from build123d import *

# Parameters (mm, degrees)
SKETCH_3_W          = 80
SKETCH_3_H          = 56
EXTRUDE_1_DEPTH     = 5
SKETCH_1_R          = 2.6
SKETCH_1_W          = 40.4
SKETCH_1_H          = 5
CUT_EXTRUDE_1_DEPTH = 5
SKETCH_5_R          = 4.85
EXTRUDE_2_DEPTH     = 4.5
FILLET_2_R          = 4


with BuildPart() as part:
    # 草图3 → 凸台-拉伸1 (new body)
    with BuildSketch(Plane(origin=(0, 0, 0), x_dir=(1, 0, 0), z_dir=(0, 1, 0))):
        Rectangle(SKETCH_3_W, SKETCH_3_H)
    extrude(amount=EXTRUDE_1_DEPTH)

    # 草图1 → 切除-拉伸1 (cut)
    with BuildSketch(Plane(origin=(0, 0, 0), x_dir=(1, 0, 0), z_dir=(0, 1, 0))):
        with Locations(Location((-31.75, 20.6375, 0), (0, 0, 90))):
            Circle(SKETCH_1_R)
        with Locations(Location((31.75, 20.6375, 0), (0, 0, 90))):
            Circle(SKETCH_1_R)
        with Locations(Location((31.75, -20.6375, 0), (0, 0, 90))):
            Circle(SKETCH_1_R)
        with Locations(Location((-31.75, -20.6375, 0), (0, 0, 90))):
            Circle(SKETCH_1_R)
        with Locations((0, -10)):
            Rectangle(SKETCH_1_W, SKETCH_1_H)
        with Locations((0, 10)):
            Rectangle(SKETCH_1_W, SKETCH_1_H)
    extrude(amount=CUT_EXTRUDE_1_DEPTH, mode=Mode.SUBTRACT)

    # 草图5 → 凸台-拉伸2 (add)
    with BuildSketch(Plane.XZ):
        with Locations(Location((31.75, 20.6375, 0), (0, 0, 270))):
            Circle(SKETCH_5_R)
    extrude(amount=EXTRUDE_2_DEPTH)

    # 圆角2
    fillet_2_edges = [part.edges().sort_by_distance(p)[0] for p in [
        (40, 2.5, 28),
        (-40, 2.5, 28),
        (-40, 2.5, -28),
        (40, 2.5, -28),
    ]]
    fillet(fillet_2_edges, radius=FILLET_2_R)


solid = part.part
Could you check a few things on this model? Use its own coordinates, in mm. A direction names the side the tool comes from. Coordinates: 2 decimals unless noted, no trailing zeros. Order: outer loops, then holes, each group sorted by start corner. A loop starts at its lowest first (then second) coordinate and runs counter-clockwise, first axis right, second up. Notation, with made-up numbers: (-37.75, -33.5) -> (-28.75, -33.5) arc R25 ccw to (-28.75, -18.5) -> close; hole circle Ø6 at (38.5, -30). An arc over 180 degrees is marked (long way). One line per item, written item: value. Start each with the question number.
1) Imagine slicing it at B-B on z = -9. List the corners of the cut face in (x, y) for me.
2) Imagine slicing it at D-D on x = 31.75. List the corners of the cut face in (y, z) for me, plus the area to 3 significant figures.
3) Imagine slicing it at C-C on y = 2.75. List the corners of the cut face in (x, z) for me, plus the area to 3 significant figures.
4) We'd pull the mould along Z, two halves only. Please class faces 4 (the flat face through (-1, 5, 0)), 5 (the flat face through (-1, 2, -28)), 6 (the flat face through (-1, 2, 28)), 7 (the flat face through (20.2, 2, -10)): +Z half, -Z half, draft (parallel to the pull), parting line (faces both ways), or undercut.
5) If I drill on L1, parallel to Z at x = 31.75, y = 2.1; L2, parallel to Z at x = 4.5, y = 1; L3, parallel to X at y = 0.5, z = -10, over which ranges is the centre line in solid material (lowest first)? Write a range as [from, to].
6) Which directions (+Z, -Z, +X, -X, +Y, -Y) give clear straight access to the entire face, cutting with the end or side of a thin tool? Please do faces 1 (the cylindrical face through (-38.859, 2.535, 26.797)), 2 (the flat face through (0, 2, -7.5)), 3 (the cylindrical face through (29.172, 2.465, 20.976)).
7) I'm going to push flat-ended pins straight in: pin 1 (1.5 mm diameter, centred on y = -1, z = 18, fed in from +X); pin 2 (1.5 mm diameter, centred on x = 22.5, z = 6.5, fed in from -Y); pin 3 (1 mm diameter, centred on y = -2, z = -1, fed in from +X). Where does each tip first touch, or does it pass through?
8) Imagine slicing it at A-A on x = -31.75. List the corners of the cut face in (y, z) for me, plus the area to 3 significant figures.
Answer list:
1. outline: (-40, 0) -> (-20.2, 0) -> (-20.2, 5) -> (-40, 5) -> close; (20.2, 0) -> (40, 0) -> (40, 5) -> (20.2, 5) -> close
2. outline: (-4.5, 15.79) -> (0, 15.79) -> (0, -18.04) -> (5, -18.04) -> (5, 18.04) -> (0, 18.04) -> (0, 23.24) -> (5, 23.24) -> (5, 28) -> (0, 28) -> (0, 25.49) -> (-4.5, 25.49) -> close; (0, -28) -> (5, -28) -> (5, -23.24) -> (0, -23.24) -> close
2. area: 272 mm2
3. outline: (-40, -24) arc R4 ccw to (-36, -28) -> (36, -28) arc R4 ccw to (40, -24) -> (40, 24) arc R4 ccw to (36, 28) -> (-36, 28) arc R4 ccw to (-40, 24) -> close; hole circle Ø5.2 at (-31.75, -20.64); hole circle Ø5.2 at (-31.75, 20.64); hole (-20.2, -12.5) -> (20.2, -12.5) -> (20.2, -7.5) -> (-20.2, -7.5) -> close; hole (-20.2, 7.5) -> (20.2, 7.5) -> (20.2, 12.5) -> (-20.2, 12.5) -> close; hole circle Ø5.2 at (31.75, -20.64); hole circle Ø5.2 at (31.75, 20.64)
3. area: 3,980 mm2
4. face 4: draft
4. face 5: -Z half
4. face 6: +Z half
4. face 7: undercut
5. L1: z = [-28, -23.24], [-18.04, 18.04], [23.24, 28]
5. L2: z = [-28, -12.5], [-7.5, 7.5], [12.5, 28]
5. L3: x = [-40, -20.2], [20.2, 40]
6. face 1: +Z, -X, +Y, -Y
6. face 2: +Y, -Y
6. face 3: +Y
7. pin 1: stops at x = 36.22
7. pin 2: stops at y = 0
7. pin 3: passes through
8. outline: (0, -28) -> (5, -28) -> (5, -23.24) -> (0, -23.24) -> close; (0, -18.04) -> (5, -18.04) -> (5, 18.04) -> (0, 18.04) -> close; (0, 23.24) -> (5, 23.24) -> (5, 28) -> (0, 28) -> close
8. area: 228 mm2
